Geometry check sheet. Reference: the model listing, model coordinates, mm. A direction names the side the tool comes from. Coordinates: 2 decimals unless noted, no trailing zeros. Order: outer loops, then holes, each group sorted by start corner. A loop starts at its lowest first (then second) coordinate and runs counter-clockwise, first axis right, second up. Notation, with made-up numbers: (74.25, 72.5) - (108.25, 72.5) arc R21 cw to (108.25, 100.5) - close; hole circle Ø3 at (29, 29.25). An arc over 180 degrees is marked (long way). Put each result on its own line as item: value.
from build123d import *

# Parameters (mm, degrees)
F0_R     = 6.1654664674
F1_DEPTH = 117.094
F2_R     = 8.4528335809
F3_DEPTH = 22.86
F5_DEPTH = 25.4


with BuildPart() as f1:
    # F0 (on Top) → F1 (new body)
    with BuildSketch(Plane.XY):
        Circle(F0_R)
    extrude(amount=F1_DEPTH)

    # F2 (on Top) → F3 (join)
    with BuildSketch(Plane.XY):
        Circle(F2_R)
    extrude(amount=F3_DEPTH)

    # F4 (on face) → F5 (join)
    with BuildSketch(Plane.XY.offset(117.094)):
        Polygon((-15.1460403576, 0), (0, 0), (0, 32.9593867064), align=None)
        Polygon((0, -22.0521092415), (0, 0), (-15.1460403576, 0), align=None)
        Polygon((0, 32.9593867064), (0, 0), (18.0666185915, 0), align=None)
        Polygon((18.0666185915, 0), (0, 0), (0, -22.0521092415), align=None)
        Polygon((-15.1460403576, 0), (0, 32.9593867064), (-15.1460403576, 32.9593867064), align=None)
    extrude(amount=F5_DEPTH)


solid = f1.part
Q1. Section check A-A on z = 130. Record the boundary of the cut face in (x, y), then the cut area to 3 significant figures.
Answer block:
outline: (-15.15, 0) - (0, -22.05) - (18.07, 0) - (0, 32.96) - (-15.15, 32.96) - close
area: 1,160 mm^2
Q2. Thickness scan on L1, parallel to Z at x = -7, y = -11.5; L2, parallel to Y at x = 0.5, z = 96.5. Record the ranges inside material, lowest first. Write a range as [from, to].
Answer block:
L1: z = [117.09, 142.49]
L2: y = [-6.15, 6.15]
Q3. Section check B-B on x = -13. Record the boundary of the cut face in (y, z), then the cut area to 3 significant figures.
Answer block:
outline: (-3.12, 117.09) - (32.96, 117.09) - (32.96, 142.49) - (-3.12, 142.49) - close
area: 917 mm^2
Q4. Section check D-D on z = 66. Record the boundary of the cut face in (x, y), then the cut area to 3 significant figures.
Answer block:
outline: circle Ø12.33 at (0, 0)
area: 119 mm^2
Q5. Depth check by flat-ended pin: pin 1 Ø2 at (x, z) = (0.5, 97.5) entering from -Y; pin 2 Ø8 at (x, z) = (10.5, 114.5) entering from +Y; pin 3 Ø10 at (x, z) = (-10.5, 97.5) entering from -Y. Enter the tip coordinate at first touch or a pass-through.
Answer block:
pin 1: stops at y = -6.17
pin 2: stops at y = 19.36
pin 3: stops at y = -2.79
Q6. Access from +Z, -Z, +X, -X, +Y, -Y to the whole of each face (thin tool, end or side, straight path). Record for faces 1 (the flat face through (-7, 32.959, 130)), 2 (the cylindrical face through (8.062, 2.539, 11.27)).
Answer block:
face 1: +Z, -Z, +X, -X, +Y
face 2: -Z
Q7. Draft check along Z on faces 3 (the flat face through (-4, -5, 22.86)), 4 (the flat face through (8.907, -11.18, 129.616)), 5 (the flat face through (0, 0, 0)), 6 (the cylindrical face through (-6.16, 0.27, 69.32)). Enter one of: pulls with the +Z half, pulls with the -Z half, needs draft (parallel to the pull), parting line crosses it, or undercut.
Answer block:
face 3: undercut
face 4: needs draft
face 5: pulls with the -Z half
face 6: undercut
Q8. Section check C-C on y = 25. Record the boundary of the cut face in (x, z), then the cut area to 3 significant figures.
Answer block:
outline: (-15.15, 117.09) - (4.36, 117.09) - (4.36, 142.49) - (-15.15, 142.49) - close
area: 496 mm^2
